The drawing under review shows one solid part. Ordinate dimensions are in mm from its lowest x, y, z. Coordinates: 2 decimals unless noted, no trailing zeros. Write each loop counter-clockwise with the first axis right and the second up, starting at its lowest first coordinate (ties: lowest second). Pieces come first, ordered by that corner, then holes. Notation, with made-up numbers: (-11, 63.25) - (45, 63.25) arc R14 ccw to (45, 87.25) - close; hole circle Ø10 at (0.5, 11.5). An arc over 180 degrees is marked (long way). Use a Markdown table: item, result.
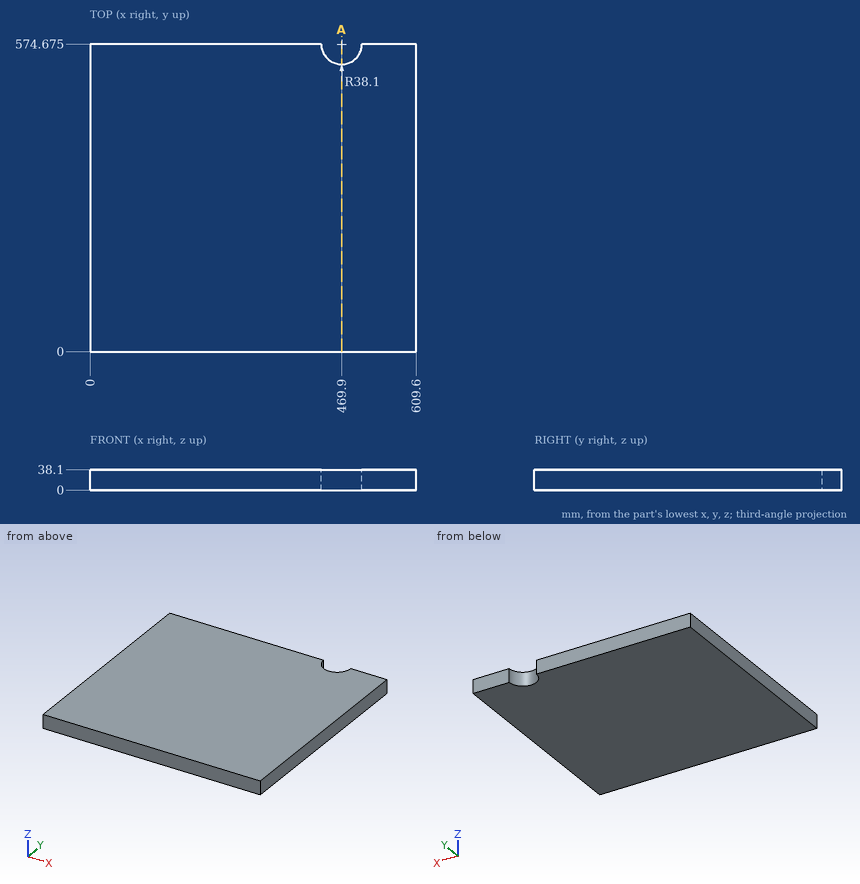
(1) For L1, parallel to Y at x = 500.5, z = 23; L2, parallel to Y at x = 447, z = 18.5, list the stretches that pass through material, from the lowest coordinate up. Write a range as from..to.
Determined:
| item | result |
|---|---|
| L1 | 0..551.98 |
| L2 | 0..544.23 |
(2) Take a section at A-A on x = 469.9. Write out the cut boundary in (y, z) (3 decimals), and give its area (3 significant figures).
Determined:
| item | result |
|---|---|
| outline | (0, 0) - (536.575, 0) - (536.575, 38.1) - (0, 38.1) - close |
| area | 20,400 mm2 |
(3) For pin 1 (12 mm diameter, centred on x = 496, z = 23, fed in from +Y), flat-tipped, find the tip position at first contact; note if it passes through.
Determined:
| item | result |
|---|---|
| pin 1 | y = 554.15 |
